Part model, mm, in its own coordinate system. A direction names the side the tool comes from. Coordinates: 2 decimals unless noted, no trailing zeros. Loops run counter-clockwise (first coordinate to the right, second up) from the corner with the lowest first, then second, coordinate; pieces in that order, holes last. Notation, with made-up numbers: M 45.25,47.25 L 50.25,47.25 A20 cw 50.25,58.25 Z; hole C -26.5,69.5 d11. An arc over 180 degrees is marked long. Use a Markdown table: item, result. Add a question column.
1) Band-saw the part on B-B (x = 20). List the corners of the cut face in (y, z), plus the area to 3 significant figures.
2) Wall check: probe 1 along X at (y, z) = (11.25, 4.5); probe 2 along X at (y, z) = (11, 12.7); probe 3 along Z at (x, y) = (14.5, 7). Give the ranges that are in metal, low to high. Write a range as from..to.
3) Band-saw the part on A-A (y = 1.75). List the corners of the cut face in (x, z) (1 decimal).
4) Band-saw the part on C-C (z = 22.25). List the corners of the cut face in (x, y).
5) Pull direction X, two halves, no side cores. Call faces 1 (the cylindrical face through (13.56, 18.99, 6.08)), 2 (the flat face through (-23.812, 8, 16)), 3 (the cylindrical face through (-13.56, 6.11, 18.99)), 4 (the flat face through (-0.333, 13.21, 16.965)): released by +X, released by -X, zero draft, split by the parting line, or undercut.
6) Band-saw the part on D-D (x = 10). List the corners of the cut face in (y, z).
7) Pin check, flat tips, straight feed: pin 1 Ø1 at (x, y) = (11, 4.5) entering from +Z; pin 2 Ø4.5 at (x, z) = (-6.5, 14.5) entering from +Y; pin 3 Ø3 at (x, y) = (17.5, 7.5) entering from +Z. Stop position of each tip, or through.
8) Tool access for faces 5 (the cylindrical face through (14.14, 7.17, 2.42)), 6 (the cylindrical face through (11.84, 6.11, 18.99)): list every direction of +Z, -Z, +X, -X, +Y, -Y with a clear straight run to the whole face (end or side of a thin tool).
from build123d import *

# Parameters (mm, degrees)
BOSS_EXTRUDE1_START     = -20.6248
BOSS_EXTRUDE1_OUTLINE_W = 47.625
BOSS_EXTRUDE1_OUTLINE_H = 20.6248
BOSS_EXTRUDE1_DEPTH     = 25.4
BOSS_EXTRUDE1_2_DEPTH   = 4.7752
BOSS_EXTRUDE1_START_2   = 4.7752
BOSS_EXTRUDE1_3_DEPTH   = 20.6248
BOSS_EXTRUDE1_START_3   = -23.8125
BOSS_EXTRUDE1_4_DEPTH   = 47.625
SKETCH2_W               = 47.625
SKETCH2_H               = 25.4
BOSS_EXTRUDE2_DEPTH     = 4.7752
FILLET1_R               = 4.7752
CUT_EXTRUDE1_DEPTH      = 60.652834174
CHAMFER2_SIZE           = 6.35
SKETCH4_R               = 4.7625
CUT_EXTRUDE2_DEPTH      = 39.181153396
SKETCH5_R               = 4.7625
CUT_EXTRUDE3_DEPTH      = 38.556588562


with BuildPart() as part:
    # Boss-Extrude1: read off the stored shape, not the designer's step
    # Boss-Extrude1 outline → Boss-Extrude1 (new body)
    with BuildSketch(Plane.XZ.offset(-4.7752).offset(BOSS_EXTRUDE1_START)):
        with Locations((0, 15.0876)):
            Rectangle(BOSS_EXTRUDE1_OUTLINE_W, BOSS_EXTRUDE1_OUTLINE_H)
        with BuildLine():
            ThreePointArc((-18.972513521, 11.711023698), (-12.7, 19.05), (-6.427486479, 11.711023698))
            ThreePointArc((-6.427486479, 11.711023698), (-12.7, 6.35), (-18.972513521, 11.711023698))
        make_face(mode=Mode.SUBTRACT)
        with BuildLine():
            ThreePointArc((6.427486479, 11.711023698), (12.7, 19.05), (18.972513521, 11.711023698))
            ThreePointArc((18.972513521, 11.711023698), (12.7, 6.35), (6.427486479, 11.711023698))
        make_face(mode=Mode.SUBTRACT)
    extrude(amount=BOSS_EXTRUDE1_DEPTH)

    # Boss-Extrude1 2 outline → Boss-Extrude1 2 (add)
    with BuildSketch(Plane.XZ.offset(-4.7752)):
        with BuildLine():
            ThreePointArc((-18.972513521, 11.711023698), (-12.7, 6.35), (-6.427486479, 11.711023698))
            ThreePointArc((-6.427486479, 11.711023698), (-12.7, 19.05), (-18.972513521, 11.711023698))
        make_face()
        with BuildLine():
            ThreePointArc((6.427486479, 11.711023698), (12.7, 6.35), (18.972513521, 11.711023698))
            ThreePointArc((18.972513521, 11.711023698), (12.7, 19.05), (6.427486479, 11.711023698))
        make_face()
    extrude(amount=BOSS_EXTRUDE1_2_DEPTH)

    # Boss-Extrude1 3 outline → Boss-Extrude1 3 (cut)
    with BuildSketch(Plane.XY.offset(BOSS_EXTRUDE1_START_2)):
        with BuildLine():
            ThreePointArc((18.972513521, 11.711023698), (12.7, 19.05), (6.427486479, 11.711023698))
            ThreePointArc((6.427486479, 11.711023698), (12.7, 6.35), (18.972513521, 11.711023698))
        make_face()
        with BuildLine():
            ThreePointArc((-6.427486479, 11.711023698), (-12.7, 19.05), (-18.972513521, 11.711023698))
            ThreePointArc((-18.972513521, 11.711023698), (-12.7, 6.35), (-6.427486479, 11.711023698))
        make_face()
    extrude(amount=BOSS_EXTRUDE1_3_DEPTH, mode=Mode.SUBTRACT)

    # Boss-Extrude1 4 outline → Boss-Extrude1 4 (cut)
    with BuildSketch(Plane.YZ.offset(BOSS_EXTRUDE1_START_3)):
        Polygon((25.4, 25.4), (4.7752, 25.4), (25.4, 4.7752), align=None)
        Polygon((4.7752, 4.7752), (18.646847397, 4.7752), (4.7752, 18.646847397), align=None)
    extrude(amount=BOSS_EXTRUDE1_4_DEPTH, mode=Mode.SUBTRACT)

    # Sketch2 → Boss-Extrude2 (add)
    with BuildSketch(Plane(origin=(0, 0, 4.7752), x_dir=(-1, 0, 0), z_dir=(0, 0, -1))):
        with Locations((0, 12.7)):
            Rectangle(SKETCH2_W, SKETCH2_H)
    extrude(amount=BOSS_EXTRUDE2_DEPTH)

    # Fillet1
    fillet1_edges = [part.edges().sort_by_distance(p)[0] for p in [
        (0, 25.4, 4.7752),
        (0, 4.7752, 25.4),
    ]]
    fillet(fillet1_edges, radius=FILLET1_R)

    # Sketch3 → Cut-Extrude1 (cut, through all)
    with BuildSketch(Plane(origin=(23.8125, 0, 0), x_dir=(0, 0, -1), z_dir=(1, 0, 0))):
        Polygon((0, 20.447), (-11.476191114, 20.447), (-2.66042984, 31.108635465), (0, 31.108635465), align=None)
    extrude(amount=-CUT_EXTRUDE1_DEPTH, mode=Mode.SUBTRACT)

    # Chamfer2
    chamfer2_edges = [part.edges().sort_by_distance(p)[0] for p in [
        (0, 20.447, 0),
    ]]
    chamfer(chamfer2_edges, length=CHAMFER2_SIZE - 0.0001)  # a hair under: the kernel refuses the full size

    # Sketch4 → Cut-Extrude2 (cut, through all)
    with BuildSketch(Plane(origin=(0, 4.7752, 0), x_dir=(1, 0, 0), z_dir=(0, 1, 0))):
        with Locations(Location((-12.7, -11.71067, 0), (0, 0, 270))):
            Circle(SKETCH4_R)
        with Locations(Location((12.7, -11.71067, 0), (0, 0, 90))):
            Circle(SKETCH4_R)
    extrude(amount=-CUT_EXTRUDE2_DEPTH, mode=Mode.SUBTRACT)

    # Sketch5 → Cut-Extrude3 (cut, through all)
    with BuildSketch(Plane.XY.offset(4.7752)):
        with Locations((-12.7, 11.71067)):
            Circle(SKETCH5_R)
        with Locations(Location((12.7, 11.71067, 0), (0, 0, 30.070595226))):
            Circle(SKETCH5_R)
    extrude(amount=-CUT_EXTRUDE3_DEPTH, mode=Mode.SUBTRACT)


solid = part.part
Entries:
| question | item | result |
|---|---|---|
| 1 | outline | M 0,0 L 14.1,0 L 20.45,6.35 L 20.45,9.73 L 6.17,24 A4.78 ccw 2.8,25.4 L 0,25.4 Z; hole M 4.78,4.78 L 18.65,4.78 L 4.78,18.65 Z |
| 1 | area | 280 mm2 |
| 2 | probe 1 | -23.81..-17.44, -7.96..7.96, 17.44..23.81 |
| 2 | probe 2 | -23.81..-19.05, -6.35..6.35, 19.05..23.81 |
| 2 | probe 3 | 0..4.78 |
| 3 | outline | M -23.8,0 L 23.8,0 L 23.8,25.4 L -23.8,25.4 Z; hole C -12.7,11.7 d9.5; hole C 12.7,11.7 d9.5 |
| 4 | outline | M -23.81,0 L 23.81,0 L 23.81,7.93 L 16.89,7.93 A6.35 cw 8.51,7.93 L -8.51,7.93 A6.35 cw -16.89,7.93 L -23.81,7.93 Z |
| 5 | face 1 | undercut |
| 5 | face 2 | released by -X |
| 5 | face 3 | undercut |
| 5 | face 4 | zero draft |
| 6 | outline | M 0,0 L 7.79,0 L 7.79,4.78 L 4.78,4.78 L 4.78,7.79 L 0,7.79 Z; M 0,15.63 L 4.78,15.63 L 4.78,18.65 L 4.97,18.45 L 6.95,18.45 L 6.95,23.22 L 6.17,24 A4.78 ccw 2.8,25.4 L 0,25.4 Z; M 15.63,1.54 L 20.45,6.35 L 20.45,6.95 L 18.45,6.95 L 18.45,4.97 L 18.65,4.78 L 15.63,4.78 Z |
| 7 | pin 1 | z = 25.25 |
| 7 | pin 2 | y = 17.92 |
| 7 | pin 3 | z = 24.17 |
| 8 | face 5 | +Z, -Z |
| 8 | face 6 | +Y |
